from build123d import *

# Parameters (mm, degrees)
F0_W          = 108.5027605295
F0_H          = 31.3708260655
F1_DEPTH      = 152.4
F2_W          = 95.2637046576
F2_H          = 21.5854328126
F3_DEPTH      = 147.32
F4_R          = 5.08
F5_W          = 39.1854047775
F5_H          = 139.895003289
F6_DEPTH      = 15.6864130328
F6_DEPTH_BACK = 15.6864130328
F7_R          = 1.27
F8_W          = 38.5659714229
F8_H          = 21.5854328126
F9_DEPTH      = 152.401


with BuildPart() as f1:
    # F0 (on Top) → F1 (new body)
    with BuildSketch(Plane.XY):
        Rectangle(F0_W, F0_H)
    extrude(amount=F1_DEPTH)

    # F2 (on Top) → F3 (cut)
    with BuildSketch(Plane.XY):
        Rectangle(F2_W, F2_H)
    extrude(amount=F3_DEPTH, mode=Mode.SUBTRACT)

    # F4
    f4_edges = [f1.edges().sort_by_distance(p)[0] for p in [
        (-54.25138, 15.685413, 76.2),
        (-54.25138, -15.685413, 76.2),
        (54.25138, -15.685413, 76.2),
        (54.25138, 15.685413, 76.2),
    ]]
    fillet(f4_edges, radius=F4_R)

    # F5 (on Front) → F6 (cut, two sides)
    with BuildSketch(Plane.XZ) as f6_sk:
        with Locations((24.835858494, 77.4077717215)):
            Rectangle(F5_W, F5_H)
        with Locations((-24.835858494, 77.4077717215)):
            Rectangle(F5_W, F5_H)
    extrude(amount=-F6_DEPTH, mode=Mode.SUBTRACT)
    extrude(f6_sk.sketch, amount=F6_DEPTH_BACK, mode=Mode.SUBTRACT)

    # F7
    f7_edges = [f1.edges().sort_by_distance(p)[0] for p in [
        (5.243156, -15.685413, 77.407772),
        (5.243156, -10.792716, 77.390135),
        (-5.243156, -15.685413, 77.407772),
        (-5.243156, -10.792716, 77.390135),
        (-5.243156, 10.792716, 77.390135),
        (-5.243156, 15.685413, 77.407772),
        (5.243156, 10.792716, 77.390135),
        (5.243156, 15.685413, 77.407772),
        (44.428561, -15.685413, 77.407772),
        (44.428561, -10.792716, 77.390135),
        (44.428561, 10.792716, 77.390135),
        (44.428561, 15.685413, 77.407772),
        (-44.428561, 10.792716, 77.390135),
        (-44.428561, 15.685413, 77.407772),
        (-44.428561, -10.792716, 77.390135),
        (-44.428561, -15.685413, 77.407772),
        (-24.835858, 15.685413, 147.355273),
        (-24.835858, -15.685413, 147.355273),
        (24.835858, -15.685413, 147.355273),
        (24.835858, 15.685413, 147.355273),
    ]]
    fillet(f7_edges, radius=F7_R)

    # F8 (on Top) → F9 (cut, through all)
    with BuildSketch(Plane.XY):
        with Locations((-24.6073936578, 0)):
            Rectangle(F8_W, F8_H)
        with Locations((24.6073936578, 0)):
            Rectangle(F8_W, F8_H)
    extrude(amount=F9_DEPTH, mode=Mode.SUBTRACT)


solid = f1.part
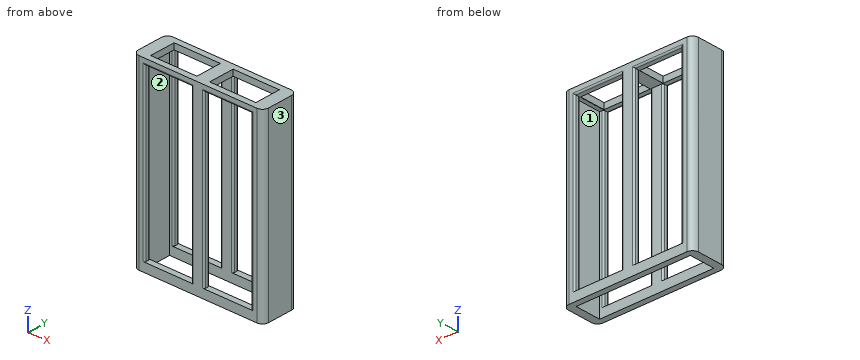
Could you check a few things on this model? Use its own coordinates, in mm. Face numbers are marked on the shaded views. Round coordinates to 2 decimals unless told otherwise and drop trailing zeros. Loops run counter-clockwise (first coordinate to the right, second up) from the corner with the lowest first, then second, coordinate; pieces in that order, holes last. Notation, with made-up numbers: (79.5, -22.5) -> (105.5, -22.5) arc R22 ccw to (105.5, 16.5) -> close; hole circle Ø1 at (-14.5, -30.75). An arc over 180 degrees is marked (long way). Use CSV: the item, a comma, the result in double quotes.
(1) Will these pins go through, and if not, where does the flat tip stop? pin 1 Ø1.6 at (x, y) = (-46.5, 2.5) entering from -Z; pin 2 Ø3 at (x, y) = (-6, -3) entering from +Z.
Return value:
pin 1,"stops at z = 147.32"
pin 2,"stops at z = 152.4"
(2) Suppose I cut it at A-A on y = -5. Give the number of separate pieces and of enclosed holes in the cut face, plus the area to 3 significant figures.
Return value:
separate pieces,"3"
enclosed holes,"0"
area,"2,110 mm²"
(3) If we mould it in two halves opening along Y, with no side actions, what happens to the marked faces 1, 2 and 3? For each: +Y half, -Y half, draft (parallel to the pull), parting line (faces both ways), or undercut.
Return value:
face 1,"undercut"
face 2,"undercut"
face 3,"draft"
(4) Suppose I cut it at B-B on x = -33.5. Write out the boundary of the cut face in (y, z), plus the area to 3 significant figures.
Return value:
outline,"(-15.69, 0) -> (-10.79, 0) -> (-10.79, 7.46) -> (-15.69, 7.46) -> close; (-15.69, 148.63) arc R1.27 ccw to (-14.42, 147.36) -> (-10.79, 147.36) -> (-10.79, 152.4) -> (-15.69, 152.4) -> close; (10.79, 0) -> (15.69, 0) -> (15.69, 7.46) -> (10.79, 7.46) -> close; (10.79, 147.36) -> (14.42, 147.36) arc R1.27 ccw to (15.69, 148.63) -> (15.69, 152.4) -> (10.79, 152.4) -> close"
area,"122 mm²"
(5) If I drill on probe 1 along X at (y, z) = (-8.5, 116.5); probe 2 along Z at (x, y) = (28.5, -11); probe 3 along X at (y, z) = (-14, 60), over which ranges is the centre line in solid material (lowest first)? Write a range as [from, to].
Return value:
probe 1,"x = [-54.25, -47.63], [47.63, 54.25]"
probe 2,"z = [0, 7.46], [147.36, 152.4]"
probe 3,"x = [-52.95, -44.43], [-5.24, 5.24], [44.43, 52.95]"
(6) Suppose I cut it at C-C on x = 0. Write out the boundary of the cut face in (y, z).
Return value:
outline,"(-15.69, 0) -> (-10.79, 0) -> (-10.79, 147.32) -> (10.79, 147.32) -> (10.79, 0) -> (15.69, 0) -> (15.69, 152.4) -> (-15.69, 152.4) -> close"
